```python
from build123d import *

# Parameters (mm, degrees)
PAD_DEPTH       = 43
SKETCH001_R     = 11.5
SKETCH001_R_2   = 1.8
POCKET_DEPTH    = 83.001
SKETCH002_R     = 1.2
POCKET001_DEPTH = 3.5


with BuildPart() as part:
    # Sketch → Pad (new body)
    with BuildSketch(Plane.XY):
        Polygon((-18.5, 3.5), (-3.5, 3.5), (-3.5, 83), (0, 83), (0, 44), (43, 44), (43, 40.5), (0, 40.5), (0, 0), (-18.5, 0), align=None)
    extrude(amount=PAD_DEPTH)

    # Sketch001 → Pocket (cut, through all)
    with BuildSketch(Plane.XZ):
        with Locations((21.15, 21.15)):
            Circle(SKETCH001_R)
        with Locations((5.65, 36.65)):
            Circle(SKETCH001_R_2)
        with Locations((36.65, 36.65)):
            Circle(SKETCH001_R_2)
        with Locations((36.65, 5.65)):
            Circle(SKETCH001_R_2)
        with Locations((5.65, 5.65)):
            Circle(SKETCH001_R_2)
        with Locations((-8.85, 31.15)):
            Circle(SKETCH001_R_2)
        with Locations((-8.85, 11.15)):
            Circle(SKETCH001_R_2)
    extrude(amount=-POCKET_DEPTH, mode=Mode.SUBTRACT)

    # Sketch002 → Pocket001 (cut)
    with BuildSketch(Plane.YZ):
        with Locations((78, 24.75)):
            Circle(SKETCH002_R)
        with Locations((78, 18.25)):
            Circle(SKETCH002_R)
    extrude(amount=-POCKET001_DEPTH, mode=Mode.SUBTRACT)


solid = part.part
```
Work out the finished part from the listing and answer in its coordinate system (mm). A direction names the side the tool comes from. Round coordinates to 2 decimals unless told otherwise and drop trailing zeros. Write each loop counter-clockwise with the first axis right and the second up, starting at its lowest first coordinate (ties: lowest second). Pieces come first, ordered by that corner, then holes.
1) A cutting plane is placed at C-C on z = 14. Determine the outline of the cut face in (x, y), and give its area (3 significant figures).
2) Consider probe 1 along Z at (x, y) = (-2, 78); probe 2 along Z at (x, y) = (-8.85, 1.35); probe 3 along X at (y, z) = (1, 31). Determine where each line is inside the solid, lowest interval first.
3) A cutting plane is placed at D-D on x = 27.5. Determine the outline of the cut face in (y, z).
4) Flat-ended cylindrical pins translate along their axes: P1, Ø12, axis at y = 20, z = 21, coming from the +X side; P2, Ø12, axis at x = 23.5, z = 10.5, coming from the +Y side; P3, Ø8, axis at x = 6.5, z = 35.5, coming from the -Y side; P4, Ø1.5, axis at x = -2, z = 22.5, coming from the -Y side. Find the tip coordinate at first contact, or state that the pin passes through.
5) A cutting plane is placed at B-B on x = -8.85. Determine the outline of the cut face in (y, z), and give its area (3 significant figures).
6) A cutting plane is placed at A-A on z = 36.65. Determine the outline of the cut face in (x, y), and give its area (3 significant figures).
7) Determine the mould class of faces 1 (the face through (43, 42, 21)), 2 (the face through (18.657, 42.226, 9.923)), 3 (the face through (-1.73, 79.11, 24.29)) for opening direction X: pulls with the +X half, pulls with the -X half, needs draft (parallel to the pull), parting line crosses it, or undercut.
8) Which of the six approach directions +Z, -Z, +X, -X, +Y, -Y give full straight-line access (tool end or side, diameter ignored) to faces 4 (the face through (31, 44, 31)), 5 (the face through (0, 21, 21)), 6 (the face through (-3.5, 43, 21))?
Entries:
1. outline: (-18.5, 0) - (0, 0) - (0, 40.5) - (12.14, 40.5) - (12.14, 44) - (0, 44) - (0, 83) - (-3.5, 83) - (-3.5, 3.5) - (-18.5, 3.5) - close; (30.16, 40.5) - (43, 40.5) - (43, 44) - (30.16, 44) - close
1. area: 430 mm2
2. probe 1: z = 0 to 17.05, 19.45 to 23.55, 25.95 to 43
2. probe 2: z = 0 to 9.35, 12.95 to 29.35, 32.95 to 43
2. probe 3: x = -18.5 to -10.64, -7.06 to 0
3. outline: (40.5, 0) - (44, 0) - (44, 11.56) - (40.5, 11.56) - close; (40.5, 30.74) - (44, 30.74) - (44, 43) - (40.5, 43) - close
4. P1: stops at x = 0
4. P2: stops at y = 44
4. P3: stops at y = 40.5
4. P4: stops at y = 0
5. outline: (0, 0) - (3.5, 0) - (3.5, 9.35) - (0, 9.35) - close; (0, 12.95) - (3.5, 12.95) - (3.5, 29.35) - (0, 29.35) - close; (0, 32.95) - (3.5, 32.95) - (3.5, 43) - (0, 43) - close
5. area: 125 mm2
6. outline: (-18.5, 0) - (0, 0) - (0, 40.5) - (3.85, 40.5) - (3.85, 44) - (0, 44) - (0, 83) - (-3.5, 83) - (-3.5, 3.5) - (-18.5, 3.5) - close; (7.45, 40.5) - (34.85, 40.5) - (34.85, 44) - (7.45, 44) - close; (38.45, 40.5) - (43, 40.5) - (43, 44) - (38.45, 44) - close
6. area: 468 mm2
7. face 1: pulls with the +X half
7. face 2: undercut
7. face 3: needs draft
8. face 4: +Z, -Z, +X, +Y
8. face 5: +Z, -Z, +X, -Y
8. face 6: +Z, -Z, -X, +Y
